Build history of the part. All positions in model axes, mm. Round coordinates to 2 decimals unless told otherwise and drop trailing zeros. Order: outer loops, then holes, each group sorted by start corner. A loop starts at its lowest first (then second) coordinate and runs counter-clockwise, first axis right, second up. Notation, with made-up numbers: (18.5, 4.25) -> (63.5, 4.25) arc R17 cw to (63.5, 34.25) -> close; hole circle Ø4 at (56, 36.25). An arc over 180 degrees is marked (long way). Use a Markdown table: item, result. Add a question column.
Item 1: Slice it at C-C, the plane x = -365. Give the cut face in (y, z).
Item 2: Pin check, flat tips, straight feed: pin 1 (1 mm diameter, centred on x = -51, y = -29, fed in from -Z); pin 2 (6 mm diameter, centred on y = -23, z = -21, fed in from -X); pin 3 (2 mm diameter, centred on y = -57.5, z = -2.5, fed in from -X). Stop position of each tip, or through.
Item 3: Slice it at A-A, the plane y = -34.5. Give the cut face in (x, z) (3 decimals).
Item 4: Probe L1, parallel to X at y = -3, z = -14; L2, parallel to X at y = -16, z = -20; L3, parallel to Z at x = -371, y = -17. List the from-to ranges inside material, lowest first.
Item 5: Slice it at B-B, the plane x = -234.5. Give the cut face in (y, z).
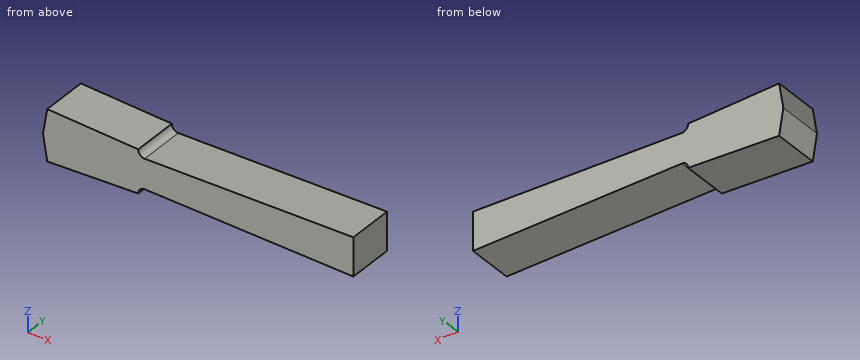
from build123d import *

# Parameters (mm, degrees)
F1_DEPTH = 69.85


with BuildPart() as f1:
    # F0 (on Front) → F1 (new body)
    with BuildSketch(Plane.XZ):
        with BuildLine():
            Line((-312.7248, -22.225), (0, -28.575))
            Line((0, -28.575), (0, 28.575))
            Line((0, 28.575), (-312.7248, 22.225))
            ThreePointArc((-312.7248, 22.225), (-319.732498, 25.092035), (-322.436157, 32.164373))
            Line((-322.436157, 32.164373), (-458.7748, 38.1))
            Line((-458.7748, 38.1), (-465.1248, 0))
            Line((-465.1248, 0), (-458.7748, -38.1))
            Line((-458.7748, -38.1), (-322.436157, -32.172233))
            ThreePointArc((-322.436157, -32.172233), (-319.735367, -25.094826), (-312.7248, -22.225))
        make_face()
    extrude(amount=F1_DEPTH)


solid = f1.part
Check sheet entries:
| question | item | result |
|---|---|---|
| 1 | outline | (-69.85, -34.02) -> (0, -34.02) -> (0, 34.02) -> (-69.85, 34.02) -> close |
| 2 | pin 1 | z = -27.55 |
| 2 | pin 2 | x = -462.12 |
| 2 | pin 3 | x = -464.87 |
| 3 | outline | (-465.125, 0) -> (-458.775, -38.1) -> (-322.436, -32.172) arc R9.527 cw to (-312.725, -22.225) -> (0, -28.575) -> (0, 28.575) -> (-312.725, 22.225) arc R9.527 cw to (-322.436, 32.164) -> (-458.775, 38.1) -> close |
| 4 | L1 | -462.79 to 0 |
| 4 | L2 | -461.79 to 0 |
| 4 | L3 | -34.28 to 34.28 |
| 5 | outline | (-69.85, -23.81) -> (0, -23.81) -> (0, 23.81) -> (-69.85, 23.81) -> close |
